Read the model definition and answer for the solid it produces. Units are mm, in the model's axes. A direction names the side the tool comes from. Coordinates: 2 decimals unless noted, no trailing zeros. Loops run counter-clockwise (first coordinate to the right, second up) from the corner with the lowest first, then second, coordinate; pieces in that order, holes last. Notation, with made-up numbers: M 5.25,-11 L 40.25,-11 A19 cw 40.25,7 Z; hole C 61.5,25 d4. An arc over 180 degrees is marked long. One line per item, written item: value. Start each with the question number.
1. Determine the mould class of faces 3 (the face through (-16.664, 0.74, 11.96)), 4 (the face through (-50.49, 0.74, -76.36)), 5 (the face through (-33, 1.5, -30)) for opening direction X: +X half, -X half, draft (parallel to the pull), parting line (faces both ways), or undercut.
2. Consider probe 1 along X at (y, z) = (0.95, -7.14); probe 2 along X at (y, z) = (1.2, -76.82); probe 3 along X at (y, z) = (0.4, -9). Determine where each line is inside the solid, lowest interval first.
3. The part is cut by section A-A (x = -49.6). Write down the section's boundary in (y, z), then the cut area to 3 significant figures.
4. The part is cut by section B-B (y = 0.35). Write down the section's boundary in (x, z), then the cut area to 3 significant figures.
5. For faces 1 (the face through (-44.6, 0.7, -47.6)), 2 (the face through (-33, 0, -30)), determine the directions among +Z, -Z, +X, -X, +Y, -Y from which every point of the face is accessible in a straight line to the end or side of a thin tool.
6. The part is cut by section C-C (z = -7.14). Write down the section's boundary in (x, y), then the cut area to 3 significant figures.
7. The part is cut by section D-D (x = -5). Write down the section's boundary in (y, z), then the cut area to 3 significant figures.
```python
from build123d import *

# Parameters (mm, degrees)
SKETCH1_R           = 1
BOSS_EXTRUDE1_DEPTH = 1.5


with BuildPart() as part:
    # Sketch1 → Boss-Extrude1 (new body)
    with BuildSketch(Plane(origin=(0, 0, 0), x_dir=(1, 0, 0), z_dir=(0, 1, 0))):
        Polygon((-33.800555393, 83.700849363), (0, 12.7), (0, 0), (-33.800555393, -24.25948244), (-53.800555393, -24.25948244), (-53.800555393, 83.700849363), align=None)
        with Locations(Location((-39.6, 76.82, 0), (0, 0, 270))):
            Circle(SKETCH1_R, mode=Mode.SUBTRACT)
        with Locations(Location((-49.6, 76.82, 0), (0, 0, 270))):
            Circle(SKETCH1_R, mode=Mode.SUBTRACT)
        with Locations(Location((-5, 7.14, 0), (0, 0, 270))):
            Circle(SKETCH1_R, mode=Mode.SUBTRACT)
        with Locations(Location((-15, 7.14, 0), (0, 0, 270))):
            Circle(SKETCH1_R, mode=Mode.SUBTRACT)
        with BuildLine():
            Line((-42.7, -14.25948244), (-42.7, 45.700849363))
            ThreePointArc((-42.7, 45.700849363), (-44.6, 47.600849363), (-46.5, 45.700849363))
            Line((-46.5, 45.700849363), (-46.5, -14.25948244))
            ThreePointArc((-46.5, -14.25948244), (-44.6, -16.15948244), (-42.7, -14.25948244))
        make_face(mode=Mode.SUBTRACT)
    extrude(amount=BOSS_EXTRUDE1_DEPTH)


solid = part.part
```
Answer block:
1. face 3: +X half
1. face 4: undercut
1. face 5: draft
2. probe 1: x = -53.8 to -46.5, -42.7 to -16, -14 to -6, -4 to 0
2. probe 2: x = -53.8 to -50.6, -48.6 to -40.6, -38.6 to -30.52
2. probe 3: x = -53.8 to -46.5, -42.7 to 0
3. outline: M 0,-83.7 L 1.5,-83.7 L 1.5,-77.82 L 0,-77.82 Z; M 0,-75.82 L 1.5,-75.82 L 1.5,24.26 L 0,24.26 Z
3. area: 159 mm2
4. outline: M -53.8,-83.7 L -33.8,-83.7 L 0,-12.7 L 0,0 L -33.8,24.26 L -53.8,24.26 Z; hole C -49.6,-76.82 d2; hole M -46.5,-45.7 A1.9 ccw -42.7,-45.7 L -42.7,14.26 A1.9 ccw -46.5,14.26 Z; hole C -39.6,-76.82 d2; hole C -15,-7.14 d2; hole C -5,-7.14 d2
4. area: 3,950 mm2
5. face 1: +Y, -Y
5. face 2: +Z, -Z, +X, -X, -Y
6. outline: M -53.8,0 L -46.5,0 L -46.5,1.5 L -53.8,1.5 Z; M -42.7,0 L -16,0 L -16,1.5 L -42.7,1.5 Z; M -14,0 L -6,0 L -6,1.5 L -14,1.5 Z; M -4,0 L 0,0 L 0,1.5 L -4,1.5 Z
6. area: 69.0 mm2
7. outline: M 0,-23.2 L 1.5,-23.2 L 1.5,-8.14 L 0,-8.14 Z; M 0,-6.14 L 1.5,-6.14 L 1.5,3.59 L 0,3.59 Z
7. area: 37.2 mm2
